Work out the finished part from the listing and answer in its coordinate system (mm). Face numbers are marked on the shaded views. A direction names the side the tool comes from. Give positions to 0.01 mm unless a question says otherwise; leave off trailing zeros. Write each loop counter-clockwise with the first axis right and the second up, starting at its lowest first coordinate (ties: lowest second). Pieces come first, ordered by that corner, then holes. Notation, with made-up numbers: (-18, 55) -> (33, 55) arc R16 ccw to (33, 77) -> close; hole circle Ø2 at (36, -19). An arc over 180 degrees is marked (long way). Use a Markdown table: item, result. Add a question column.
Q1. For a pull along Y with two mould halves and no side action, classify the marked faces 3, 4 and 5 as pulls with the +Y half, pulls with the -Y half, needs draft (parallel to the pull), parting line crosses it, or undercut.
Q2. Section D-D, the plane y = 15 is taken. Give the vertices of the cut face in (x, z), plus the area to 3 significant figures.
Q3. Section B-B, the plane z = 0 is taken. Give the vertices of the cut face in (x, y).
Q4. Section A-A, the plane y = 0 is taken. Give the vertices of the cut face in (x, z).
Q5. Consider line 1 (Z direction, x = 1.3, y = 0); line 2 (Y direction, x = 3.25, z = -0.5); line 3 (X direction, y = 5.5, z = 3.25). Determine where each line is inside the solid, lowest interval first.
Q6. For the marked faces 1 and 2, determine the directions among +Z, -Z, +X, -X, +Y, -Y from which every point of the face is accessible in a straight line to the end or side of a thin tool.
Q7. Section C-C, the plane x = 3.4 is taken. Give the vertices of the cut face in (y, z).
Q8. Each of these flat-tipped pins is pushed along its axis until it touches: pin 1 Ø2.5 at (y, z) = (15, 0) entering from +X (3 decimals); pin 2 Ø6.5 at (y, z) = (0, 0) entering from +X; pin 3 Ø5 at (y, z) = (11, -1) entering from -X; pin 4 Ø5 at (y, z) = (1, 3) entering from +X. Where does it stop, or does it pass through?
from build123d import *

# Parameters (mm, degrees)
SKETCH_1_R          = 2
SKETCH_1_R_2        = 1.5
EXTRUDE_1_DEPTH     = 5
SKETCH_2_R          = 3
SKETCH_2_R_2        = 2
EXTRUDE_2_DEPTH     = 0.5
SKETCH_3_R          = 3.5
SKETCH_3_R_2        = 2
CUT_EXTRUDE_1_DEPTH = 3


with BuildPart() as part:
    # 草图1 → 凸台-拉伸1 (new body)
    with BuildSketch(Plane(origin=(0, 0, 0), x_dir=(0, 0, -1), z_dir=(1, 0, 0))):
        with BuildLine():
            Line((-7.779174478, 1.866666667), (-4.375785644, 16.05))
            ThreePointArc((-4.375785644, 16.05), (0, 19.5), (4.375785644, 16.05))
            Line((4.375785644, 16.05), (7.779174478, 1.866666667))
            ThreePointArc((7.779174478, 1.866666667), (0, -8), (-7.779174478, 1.866666667))
        make_face()
        Circle(SKETCH_1_R, mode=Mode.SUBTRACT)
        with Locations((0, 15)):
            Circle(SKETCH_1_R_2, mode=Mode.SUBTRACT)
    extrude(amount=EXTRUDE_1_DEPTH)

    # 草图2 → 凸台-拉伸2 (add)
    with BuildSketch(Plane.ZY):
        Circle(SKETCH_2_R)
        Circle(SKETCH_2_R_2, mode=Mode.SUBTRACT)
    extrude(amount=EXTRUDE_2_DEPTH)

    # 草图3 → 切除-拉伸1 (cut)
    with BuildSketch(Plane(origin=(5, 0, 0), x_dir=(0, 0, -1), z_dir=(1, 0, 0))):
        Circle(SKETCH_3_R)
        Circle(SKETCH_3_R_2, mode=Mode.SUBTRACT)
    extrude(amount=-CUT_EXTRUDE_1_DEPTH, mode=Mode.SUBTRACT)


solid = part.part
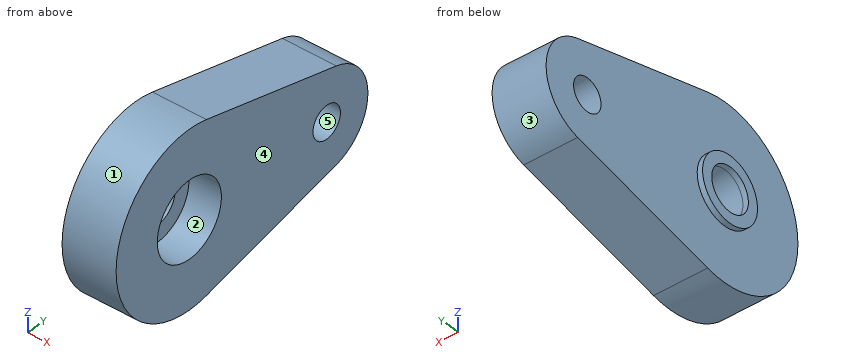
Result set:
| question | item | result |
|---|---|---|
| 1 | face 3 | pulls with the +Y half |
| 1 | face 4 | needs draft |
| 1 | face 5 | undercut |
| 2 | outline | (0, -4.63) -> (5, -4.63) -> (5, -1.5) -> (0, -1.5) -> close; (0, 1.5) -> (5, 1.5) -> (5, 4.63) -> (0, 4.63) -> close |
| 2 | area | 31.3 mm2 |
| 3 | outline | (-0.5, -3) -> (0, -3) -> (0, -8) -> (5, -8) -> (5, -3.5) -> (2, -3.5) -> (2, -2) -> (-0.5, -2) -> close; (-0.5, 2) -> (2, 2) -> (2, 3.5) -> (5, 3.5) -> (5, 13.5) -> (0, 13.5) -> (0, 3) -> (-0.5, 3) -> close; (0, 16.5) -> (5, 16.5) -> (5, 19.5) -> (0, 19.5) -> close |
| 4 | outline | (-0.5, -3) -> (0, -3) -> (0, -8) -> (5, -8) -> (5, -3.5) -> (2, -3.5) -> (2, -2) -> (-0.5, -2) -> close; (-0.5, 2) -> (2, 2) -> (2, 3.5) -> (5, 3.5) -> (5, 8) -> (0, 8) -> (0, 3) -> (-0.5, 3) -> close |
| 5 | line 1 | z = -8 to -2, 2 to 8 |
| 5 | line 2 | y = -7.98 to -3.46, 3.46 to 13.59, 16.41 to 19.47 |
| 5 | line 3 | x = 0 to 5 |
| 6 | face 1 | +X, -X |
| 6 | face 2 | +X |
| 7 | outline | (1.87, -7.78) -> (16.05, -4.38) arc R4.5 ccw to (16.05, 4.38) -> (1.87, 7.78) arc R8 ccw (long way) to start; hole circle Ø7 at (0, 0); hole circle Ø3 at (15, 0) |
| 8 | pin 1 | passes through |
| 8 | pin 2 | stops at x = 2 |
| 8 | pin 3 | stops at x = 0 |
| 8 | pin 4 | stops at x = 5 |
